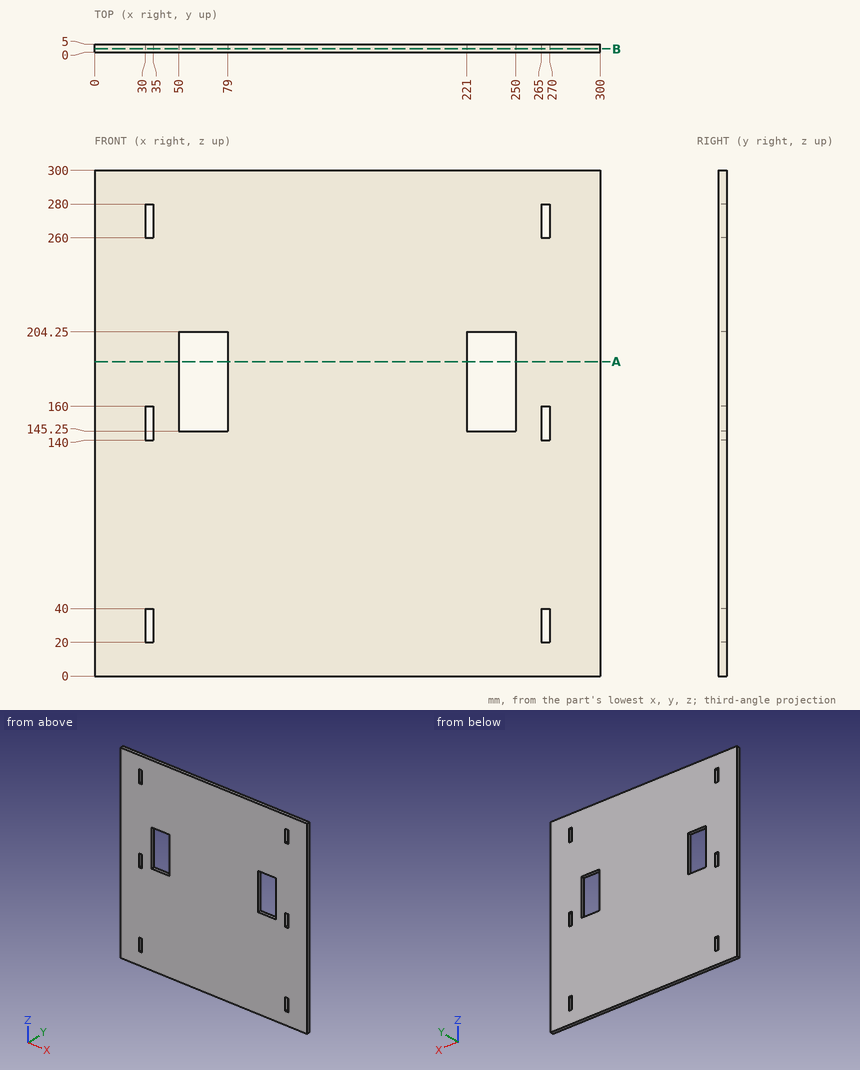
Check sheet for the drawn part. Datum: minimum x, y, z corner. Units: mm. Round coordinates to 2 decimals unless told otherwise and drop trailing zeros. Loops run counter-clockwise (first coordinate to the right, second up) from the corner with the lowest first, then second, coordinate; pieces in that order, holes last. Notation, with made-up numbers: (59, -10.75) - (95, -10.75) arc R9 cw to (95, -5.75) - close; hole circle Ø11 at (69.25, -28). An arc over 180 degrees is marked (long way). Answer as a JSON object with one key per item and string values. Group by question number.
Q1. Sectioned sample at B-B, the plane y = 2.1. Count the separate pieces of the cut face and the enclosed holes in it, plus the area to 3 significant figures.
Q2. Sectioned sample at A-A, the plane z = 186.5. Enter the section's corners in (x, y).
Q3. Gauge pin test, flat end, axial feed: P1, Ø2.5, axis at y = 2.5, z = 28.5, coming from the -X side. Record the tip position at first contact, or that the pin passes through.
Q4. Scan lines: line 1 along X through (y, z) = (3.25, 167.5); line 2 along X through (y, z) = (2.1, 267); line 3 along Z through (x, y) = (53, 3.1). Record each from-to range of solid material in increasing order. Write a range as [from, to].
Solution:
{
 "1": {"separate pieces": "1", "enclosed holes": "8", "area": "86,000 mm²"},
 "2": {"outline": "(0, 0) - (50, 0) - (50, 5) - (0, 5) - close; (79, 0) - (221, 0) - (221, 5) - (79, 5) - close; (250, 0) - (300, 0) - (300, 5) - (250, 5) - close"},
 "3": {"P1": "stops at x = 0"},
 "4": {"line 1": "x = [0, 50], [79, 221], [250, 300]", "line 2": "x = [0, 30], [35, 265], [270, 300]", "line 3": "z = [0, 145.25], [204.25, 300]"}
}
